from build123d import *

# Parameters (mm, degrees)
CHAMFER_1_SIZE = 0.15


with BuildPart() as part:
    # Эскиз1 → Повернуть1 (revolve)
    with BuildSketch(Plane.XY, mode=Mode.PRIVATE) as revolve_1_sk:
        with BuildLine():
            Line((6.4048, 12), (6.4048, 9.9286))
            ThreePointArc((6.4048, 9.9286), (6.881, 8.5), (6.4048, 7.0714))
            Line((6.4048, 7.0714), (6.4048, 5.5))
            Line((6.4048, 5.5), (8.7, 5.5))
            ThreePointArc((8.7, 5.5), (8.912132034, 5.587867966), (9, 5.8))
            Line((9, 5.8), (9, 11.7))
            ThreePointArc((9, 11.7), (8.912132034, 11.912132034), (8.7, 12))
            Line((8.7, 12), (6.4048, 12))
        make_face()
    revolve(revolve_1_sk.sketch.rotate(Axis((6.4048, 0, 0), (1, 0, 0)), 270), axis=Axis((6.4048, 0, 0), (1, 0, 0)))

    # Фаска1
    chamfer_1_edges = [part.edges().sort_by_distance(p)[0] for p in [
        (6.4048, 0, 12),
        (6.4048, 0, 5.5),
    ]]
    chamfer(chamfer_1_edges, length=CHAMFER_1_SIZE)


solid = part.part
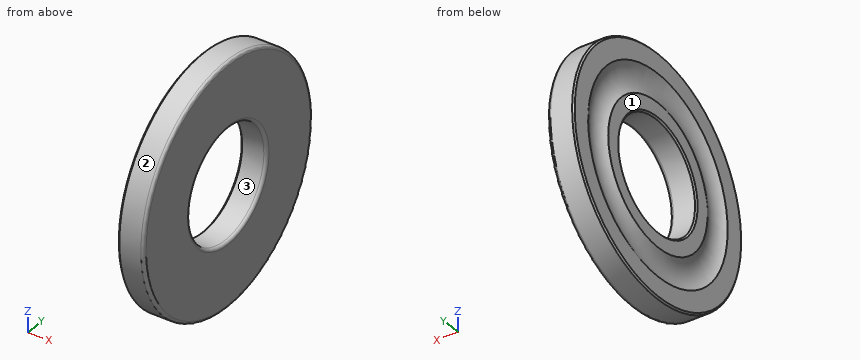
Source: CAD feature listing. Evaluate the final solid. Frame: model axes, mm. Face numbers are marked on the shaded views. Coordinates: 2 decimals unless noted, no trailing zeros. Loops run counter-clockwise (first coordinate to the right, second up) from the corner with the lowest first, then second, coordinate; pieces in that order, holes last. Notation, with made-up numbers: (77.5, 23.5) - (124.5, 23.5) arc R12 ccw to (124.5, 39.5) - close; hole circle Ø7 at (69, 13). An arc over 180 degrees is marked (long way). One line per question, with ' | ' between items.
1) Section C-C, the plane x = 7.25. Return loops of the section in (y, z), then the cut area to 3 significant figures.
Report:
outline: circle Ø24 at (0, 0); hole circle Ø11 at (0, 0) | area: 357 mm²
2) Pull-direction query (Z, two-part tool) for the marked faces 1, 2 and 3; classes: released by +Z, released by -Z, zero draft, split by the parting line, or undercut.
Report:
face 1: zero draft | face 2: split by the parting line | face 3: undercut
3) Section A-A, the plane y = 0. Return loops of the section in (x, z), then the cut area to 3 significant figures.
Report:
outline: (6.4, -11.85) - (6.55, -12) - (8.7, -12) arc R0.3 ccw to (9, -11.7) - (9, -5.8) arc R0.3 ccw to (8.7, -5.5) - (6.55, -5.5) - (6.4, -5.65) - (6.4, -7.07) arc R2.38 cw to (6.4, -9.93) - close; (6.4, 5.65) - (6.55, 5.5) - (8.7, 5.5) arc R0.3 ccw to (9, 5.8) - (9, 11.7) arc R0.3 ccw to (8.7, 12) - (6.55, 12) - (6.4, 11.85) - (6.4, 9.93) arc R2.38 cw to (6.4, 7.07) - close | area: 31.8 mm²
4) First-contact query: P1, Ø1.5, axis at x = 7, z = -0.5, coming from the +Y side; P2, Ø10, axis at y = 0, z = 0, coming from the +X side. Flat tips, straight axial feed; report the tip coordinate or a pass-through.
Report:
P1: stops at y = 12 | P2: passes through
5) Line query: line 1 along Y through (x, z) = (8.3, 0); line 2 along Y through (x, z) = (8.65, -5); line 3 along Z through (x, y) = (7.5, 2.25). Output: solid intervals per line, ascending.
Report:
line 1: y = -12 to -5.5, 5.5 to 12 | line 2: y = -10.91 to -2.29, 2.29 to 10.91 | line 3: z = -11.79 to -5.02, 5.02 to 11.79
